Check sheet for the modelled part. Datum: model origin and axes. Units: mm. Face numbers are marked on the shaded views. A direction names the side the tool comes from. Coordinates: 2 decimals unless noted, no trailing zeros. Write each loop counter-clockwise with the first axis right and the second up, starting at its lowest first coordinate (ties: lowest second). Pieces come first, ordered by that corner, then holes. Notation, with made-up numbers: (51.5, 34) - (71.5, 34) arc R24 ccw to (71.5, 49) - close; hole circle Ø10 at (47.5, 25). An arc over 180 degrees is marked (long way). Use one line per item in the form item = value. Start each with the question number.
1. Cross-section at D-D on z = 4.5. Record the boundary of the cut face in (x, y).
2. Scan lines: line 1 along Y through (x, z) = (0, 1); line 2 along Y through (x, z) = (2, 1.5); line 3 along X through (y, z) = (46.5, 1). Record each from-to range of solid material in increasing order.
3. Draft check along X on the marked faces 1, 2 and 3. Enter one of: +X half, -X half, draft (parallel to the pull), parting line (faces both ways), or undercut.
4. Go/stop test with flat-tipped pins: pin 1 Ø1.5 at (y, z) = (6, 8.5) entering from -X; pin 2 Ø1.5 at (y, z) = (11.5, 8) entering from +X; pin 3 Ø2 at (y, z) = (20, 5.5) entering from +X; pin 4 Ø2.5 at (x, z) = (2, 5.5) entering from -Y. Record where each tip stops, or that it passes through.
5. Cross-section at A-A on x = 0. Record the boundary of the cut face in (y, z).
6. Cross-section at B-B on z = 2.25. Record the boundary of the cut face in (x, y), then the cut area to 3 significant figures.
7. Tool access check on the marked faces 4, 5 and 6. Record the directions out of +Z, -Z, +X, -X, +Y, -Y that give a thin tool (end or side, any length) a straight path to the whole face; none if there is none.
8. Cross-section at C-C on y = 37. Record the boundary of the cut face in (x, z), then the cut area to 3 significant figures.
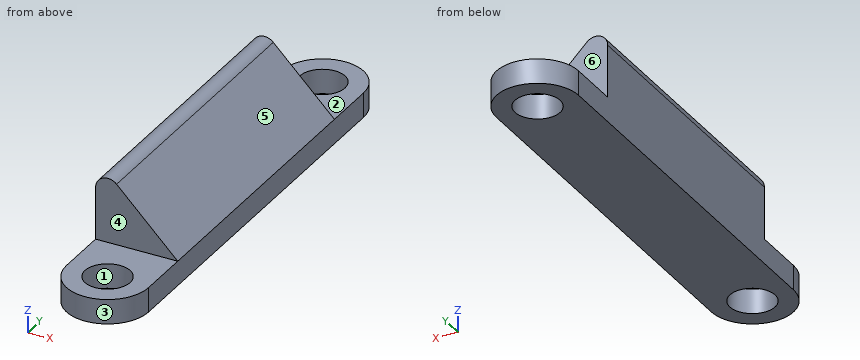
```python
from build123d import *

# Parameters (mm, degrees)
SKETCH_R     = 2.75
PAD_DEPTH    = 3
PAD001_DEPTH = 35
FILLET_R     = 1.5


with BuildPart() as part:
    # Sketch → Pad (new body)
    with BuildSketch(Plane.XY):
        with BuildLine():
            ThreePointArc((5, 48), (0, 53), (-5, 48))
            Line((-5, 48), (-5, 0))
            ThreePointArc((-5, 0), (0, -5), (5, 0))
            Line((5, 48), (5, 0))
        make_face()
        with Locations((0, 48)):
            Circle(SKETCH_R, mode=Mode.SUBTRACT)
        Circle(SKETCH_R, mode=Mode.SUBTRACT)
    extrude(amount=PAD_DEPTH)

    # Sketch001 → Pad001 (join)
    with BuildSketch(Plane.XZ.offset(-6.5)):
        Polygon((-5, 3), (-5, 13), (5, 3), align=None)
    extrude(amount=-PAD001_DEPTH)

    # Fillet
    fillet_edges = [part.edges().sort_by_distance(p)[0] for p in [
        (-5, 24, 13),
    ]]
    fillet(fillet_edges, radius=FILLET_R)


solid = part.part
```
Final values:
q1.outline = (-5, 6.5) - (3.5, 6.5) - (3.5, 41.5) - (-5, 41.5) - close
q2.line_1 = -5 to -2.75, 2.75 to 45.25, 50.75 to 53
q2.line_2 = -4.58 to -1.89, 1.89 to 46.11, 49.89 to 52.58
q2.line_3 = -5 to -2.3, 2.3 to 5
q3.face_1 = undercut
q3.face_2 = draft
q3.face_3 = parting line
q4.pin_1 = -5
q4.pin_2 = 0.75
q4.pin_3 = 3.5
q4.pin_4 = 6.5
q5.outline = (-5, 0) - (-2.75, 0) - (-2.75, 3) - (-5, 3) - close; (2.75, 0) - (45.25, 0) - (45.25, 3) - (41.5, 3) - (41.5, 8) - (6.5, 8) - (6.5, 3) - (2.75, 3) - close; (50.75, 0) - (53, 0) - (53, 3) - (50.75, 3) - close
q6.outline = (-5, 0) arc R5 ccw to (5, 0) - (5, 48) arc R5 ccw to (-5, 48) - close; hole circle Ø5.5 at (0, 0); hole circle Ø5.5 at (0, 48)
q6.area = 511 mm²
q7.face_4 = +Z, +X, -X, -Y
q7.face_5 = +Z, +X, +Y, -Y
q7.face_6 = +Z, +X, -X, +Y
q8.outline = (-5, 0) - (5, 0) - (5, 3) - (-2.44, 10.44) arc R1.5 ccw to (-5, 9.38) - close
q8.area = 77.2 mm²
